CAD build for the part. Positions are in the model's coordinates, mm. A direction names the side the tool comes from. Coordinates: 2 decimals unless noted, no trailing zeros. Order: outer loops, then holes, each group sorted by start corner. A loop starts at its lowest first (then second) coordinate and runs counter-clockwise, first axis right, second up. Notation, with made-up numbers: M 78.5,-16.75 L 114.5,-16.75 A13 cw 114.5,-7.75 Z; hole C 49,40.25 d8. An arc over 180 degrees is marked long. One line per item, written item: value.
from build123d import *

# Parameters (mm, degrees)
F1_DEPTH = 18


with BuildPart() as f1:
    # F0 (on Top) → F1 (new body)
    with BuildSketch(Plane.XY):
        Polygon((-350, -125), (-350, -157), (-300, -157), (-300, -175), (-250, -175), (-250, -157), (-200, -157), (-200, -175), (-150, -175), (-150, -157), (-100, -157), (-100, -175), (-50, -175), (-50, -157), (0, -157), (50, -157), (50, -175), (100, -175), (100, -157), (150, -157), (150, -175), (200, -175), (200, -157), (250, -157), (250, -175), (300, -175), (300, -157), (332, -157), (350, -157), (350, -125), (332, -125), (332, -75), (350, -75), (350, -25), (332, -25), (332, 25), (350, 25), (350, 75), (332, 75), (332, 125), (350, 125), (350, 157), (300, 157), (300, 175), (250, 175), (250, 157), (200, 157), (200, 175), (150, 175), (150, 157), (100, 157), (100, 175), (50, 175), (50, 157), (0, 157), (-50, 157), (-50, 175), (-100, 175), (-100, 157), (-150, 157), (-150, 175), (-200, 175), (-200, 157), (-250, 157), (-250, 175), (-300, 175), (-300, 157), (-350, 157), (-350, 125), (-332, 125), (-332, 75), (-350, 75), (-350, 25), (-332, 25), (-332, -25), (-350, -25), (-350, -75), (-332, -75), (-332, -125), align=None)
    extrude(amount=F1_DEPTH)


solid = f1.part
Q1. Slice it at A-A (x = 143.5). List the corners of the cut face in (y, z), plus the area to 3 significant figures.
Recorded:
outline: M -157,0 L 157,0 L 157,18 L -157,18 Z
area: 5,650 mm^2
Q2. Drill centre lines: line 1 along Y through (x, z) = (116.5, 4.5); line 2 along X through (y, z) = (-98, 3.25). Where is each one in solid material? Low to high.
Recorded:
line 1: y = -157 to 157
line 2: x = -332 to 332
Q3. Mould opens along Y. For faces 1 (the face through (341, 75, 9)), 2 (the face through (-275, 175, 9)), 3 (the face through (225, -157, 9)), 4 (the face through (-150, 166, 9)) say: released by +Y, released by -Y, zero draft, split by the parting line, or undercut.
Recorded:
face 1: undercut
face 2: released by +Y
face 3: released by -Y
face 4: zero draft
Q4. Slice it at B-B (y = 9.5). List the corners of the cut face in (x, z).
Recorded:
outline: M -332,0 L 332,0 L 332,18 L -332,18 Z
Q5. Pin check, flat tips, straight feed: pin 1 Ø9 at (x, z) = (345.5, 9) entering from +Y; pin 2 Ø5.5 at (y, z) = (0.5, 9) entering from +X; pin 3 Ø8 at (x, z) = (-215.5, 8.5) entering from -Y. Stop position of each tip, or through.
Recorded:
pin 1: stops at y = 157
pin 2: stops at x = 332
pin 3: stops at y = -157
Q6. Which spindle directions (+Z, -Z, +X, -X, +Y, -Y) get a long thin tool onto all of the face, cutting with end or side? Do faces 5 (the face through (-300, -166, 9)), 6 (the face through (125, 157, 9)), 7 (the face through (-125, -157, 9)), 8 (the face through (341, -25, 9)), 9 (the face through (-332, 0, 9)). Say none if no direction does.
Recorded:
face 5: +Z, -Z, -X, -Y
face 6: +Z, -Z, +Y
face 7: +Z, -Z, -Y
face 8: +Z, -Z, +X
face 9: +Z, -Z, -X
